Verification items for this drawing (mm, ordinates from the low corner). Round coordinates to 2 decimals unless told otherwise and drop trailing zeros. Order: outer loops, then holes, each group sorted by start corner. A loop starts at its lowest first (then second) coordinate and runs counter-clockwise, first axis right, second up. Notation, with made-up numbers: (64.25, 8) - (105.25, 8) arc R31 ccw to (105.25, 32) - close; hole circle Ø7 at (-16.5, 36.5). An arc over 180 degrees is marked (long way). One line per question, with ' | ' between items. Start each with the question number.
Q1. Sectioned sample at A-A, the plane y = 2.5. Enter the section's corners in (x, z) (1 decimal).
Q2. Mould release check, pull along X, two halves, no side actions. Record for the marked faces 1, 2 and 3: +X half, -X half, draft (parallel to the pull), parting line (faces both ways), or undercut.
Q3. Material ranges on line 1 along X through (y, z) = (2.5, 32.5) (1 decimal); line 2 along X through (y, z) = (5, 33) (1 decimal); line 3 along Z through (x, y) = (6.5, 2) (1 decimal), recorded low to high.
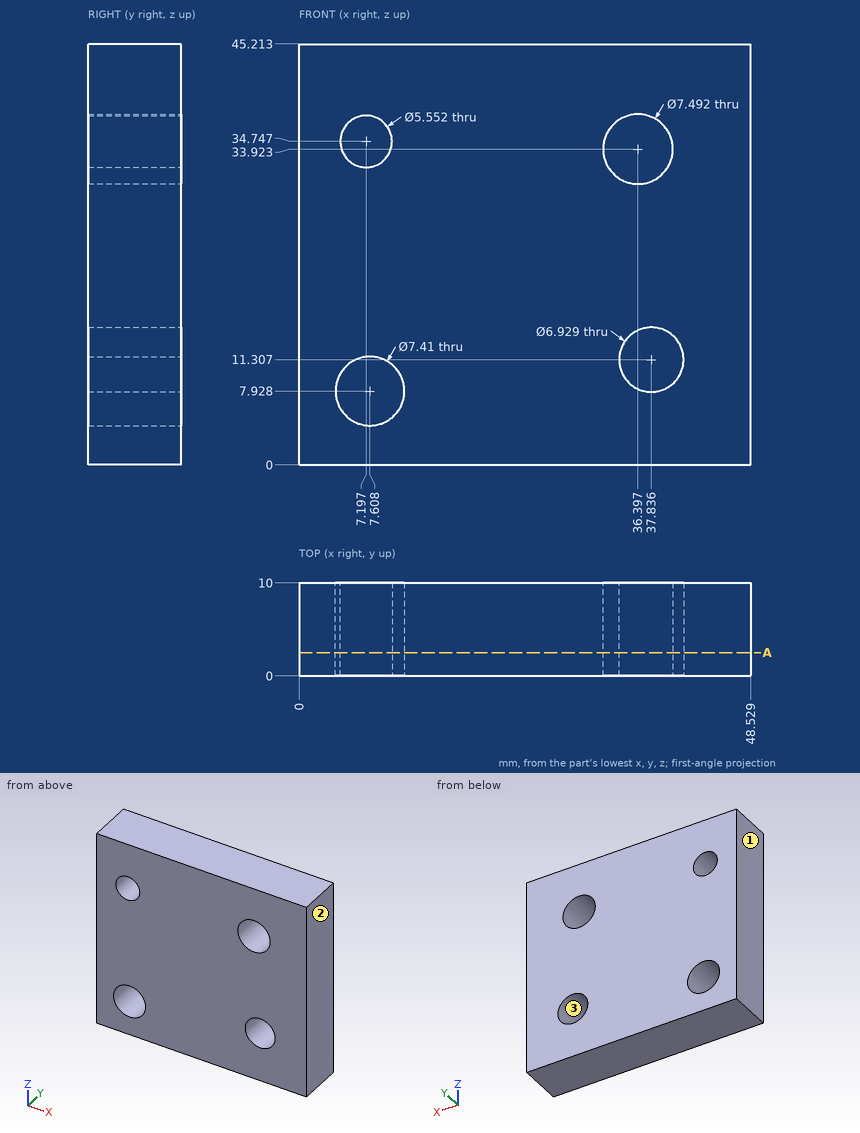
Determined:
1) outline: (0, 0) - (48.5, 0) - (48.5, 45.2) - (0, 45.2) - close; hole circle Ø7.4 at (7.6, 7.9); hole circle Ø5.6 at (7.2, 34.7); hole circle Ø7.5 at (36.4, 33.9); hole circle Ø6.9 at (37.8, 11.3)
2) face 1: -X half | face 2: +X half | face 3: undercut
3) line 1: x = 0 to 5.6, 8.8 to 32.9, 39.9 to 48.5 | line 2: x = 0 to 5, 9.4 to 32.8, 40 to 48.5 | line 3: z = 0 to 4.4, 11.5 to 32.1, 37.4 to 45.2
